Geometry: see drawing. Coordinates: mm, zero at the bounding-box minimum. Coordinates: 2 decimals unless noted, no trailing zeros. Loops run counter-clockwise (first coordinate to the right, second up) from the corner with the lowest first, then second, coordinate; pieces in that order, holes last.
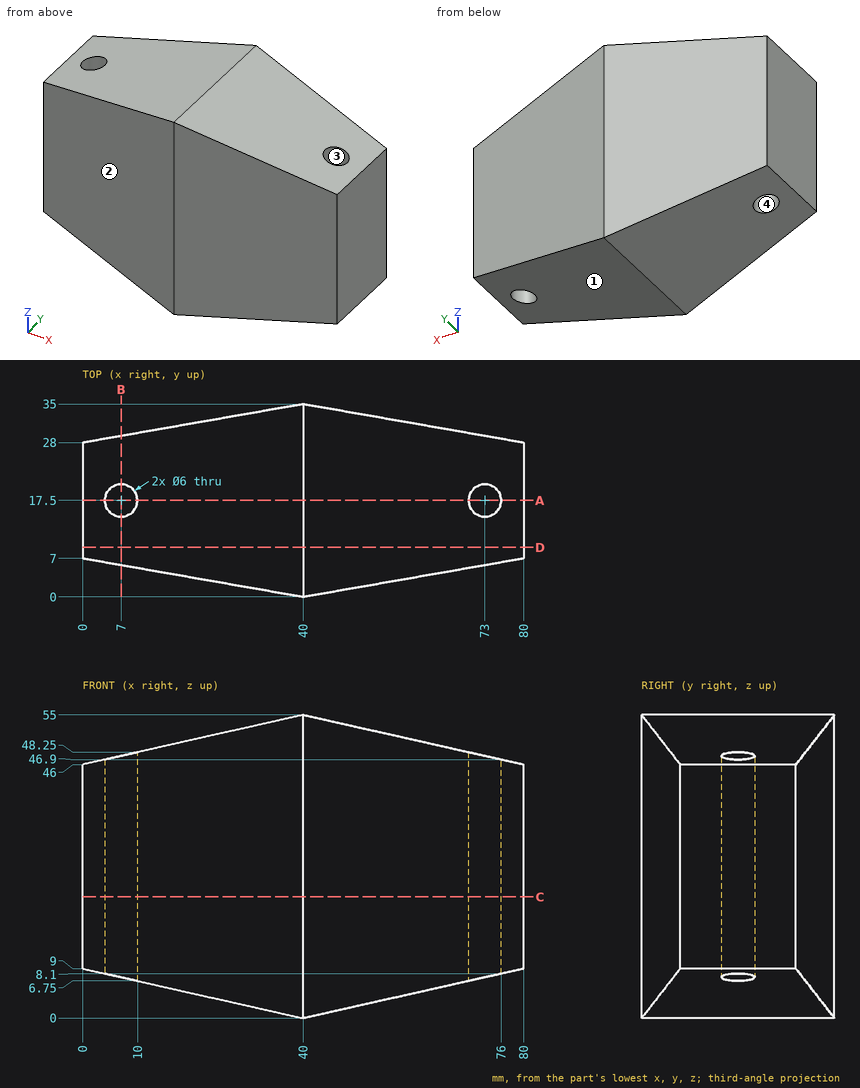
Item 1: Mould query, pull axis Y, two halves, no side actions, for the marked faces 1, 2, 3 and 4. Classes: +Y half, -Y half, draft (parallel to the pull), parting line (faces both ways), or undercut.
Result:
face 1: draft
face 2: -Y half
face 3: undercut
face 4: undercut
Item 2: Section query D-D (y = 9). Output: boundary loops of the cut face in (x, z), then the cut area to 3 significant figures.
Result:
outline: (0, 9) - (40, 0) - (80, 9) - (80, 46) - (40, 55) - (0, 46) - close
area: 3,680 mm2
Item 3: Contact query for flat-ended pins moving along their axis: P1, Ø8, axis at x = 10.5, y = 23.5, coming from the +Z side; P2, Ø8, axis at x = 59, z = 6, coming from the +Y side (3 decimals); P3, Ø8, axis at x = 19.5, y = 23.5, coming from the -Z side. Output: stop coordinate, or through.
Result:
P1: stops at z = 49.26
P2: stops at y = 32.375
P3: stops at z = 3.71
Item 4: Line query: L1, parallel to X at y = 17, z = 25; L2, parallel to X at y = 18.5, z = 29.5; L3, parallel to Y at x = 7, z = 26.5 (3 decimals). Output: solid intervals per line, ascending.
Result:
L1: x = 0 to 4.04, 9.96 to 70.04, 75.96 to 80
L2: x = 0 to 4.17, 9.83 to 70.17, 75.83 to 80
L3: y = 5.775 to 14.5, 20.5 to 29.225
Item 5: Section query B-B (x = 7). Output: boundary loops of the cut face in (y, z) (3 decimals).
Result:
outline: (5.775, 7.425) - (14.5, 7.425) - (14.5, 47.575) - (5.775, 47.575) - close; (20.5, 7.425) - (29.225, 7.425) - (29.225, 47.575) - (20.5, 47.575) - close
Item 6: Section query A-A (y = 17.5). Output: boundary loops of the cut face in (x, z), then the cut area to 3 significant figures.
Result:
outline: (0, 9) - (4, 8.1) - (4, 46.9) - (0, 46) - close; (10, 6.75) - (40, 0) - (70, 6.75) - (70, 48.25) - (40, 55) - (10, 48.25) - close; (76, 8.1) - (80, 9) - (80, 46) - (76, 46.9) - close
area: 3,200 mm2
Item 7: Section query C-C (z = 22). Output: boundary loops of the cut face in (x, y).
Result:
outline: (0, 7) - (40, 0) - (80, 7) - (80, 28) - (40, 35) - (0, 28) - close; hole circle Ø6 at (7, 17.5); hole circle Ø6 at (73, 17.5)
